```python
from build123d import *

# Parameters (mm, degrees)
SKETCH1_R           = 27.875
SKETCH1_R_2         = 17.875
BOSS_EXTRUDE1_DEPTH = 196.5
SKETCH2_R           = 11.53
CUT_EXTRUDE1_DEPTH  = 201.415271998


with BuildPart() as part:
    # Sketch1 → Boss-Extrude1 (new body)
    with BuildSketch(Plane(origin=(0, 0, 0), x_dir=(1, 0, 0), z_dir=(0, 1, 0))):
        with Locations(Location((0, 0, 0), (0, 0, 270))):
            Circle(SKETCH1_R)
        with Locations(Location((0, 0, 0), (0, 0, 270))):
            Circle(SKETCH1_R_2, mode=Mode.SUBTRACT)
    extrude(amount=BOSS_EXTRUDE1_DEPTH)

    # Sketch2 → Cut-Extrude1 (cut, through all)
    with BuildSketch(Plane(origin=(0, 0, 0), x_dir=(0, 0, -1), z_dir=(1, 0, 0))):
        with Locations((0, 131.8)):
            Circle(SKETCH2_R)
        with Locations((0, 80.8)):
            Circle(SKETCH2_R)
        with Locations((0, 29.8)):
            Circle(SKETCH2_R)
    extrude(amount=-CUT_EXTRUDE1_DEPTH, mode=Mode.SUBTRACT)


solid = part.part
```
Work out the finished part from the listing and answer in its coordinate system (mm). A direction names the side the tool comes from. Give positions to 0.01 mm unless a question says otherwise; leave off trailing zeros. Write each loop counter-clockwise with the first axis right and the second up, starting at its lowest first coordinate (ties: lowest second). Pieces come first, ordered by that corner, then holes.
(1) The part is cut by section B-B on x = 0. Write down the section's boundary in (y, z) (3 decimals).
Final values:
outline: (0, -27.875) - (196.5, -27.875) - (196.5, -17.875) - (0, -17.875) - close; (0, 17.875) - (196.5, 17.875) - (196.5, 27.875) - (0, 27.875) - close
(2) The part is cut by section D-D on z = -7.5. Write down the section's boundary in (x, y), plus the area to 3 significant figures.
Final values:
outline: (-26.85, 0) - (-16.23, 0) - (-16.23, 21.04) - (-26.85, 21.04) - close; (-26.85, 38.56) - (-16.23, 38.56) - (-16.23, 72.04) - (-26.85, 72.04) - close; (-26.85, 89.56) - (-16.23, 89.56) - (-16.23, 123.04) - (-26.85, 123.04) - close; (-26.85, 140.56) - (-16.23, 140.56) - (-16.23, 196.5) - (-26.85, 196.5) - close; (16.23, 0) - (26.85, 0) - (26.85, 196.5) - (16.23, 196.5) - close
area: 3,620 mm2
(3) Straight lines are drawn through the part: line 1 (Y direction, x = -18.75, z = 0); line 2 (X direction, y = 177, z = 1); line 3 (Z direction, x = -8.5, y = 85). For each, find the intervals that lie inside material, in ascending order.
Final values:
line 1: y = 0 to 18.27, 41.33 to 69.27, 92.33 to 120.27, 143.33 to 196.5
line 2: x = -27.86 to -17.85, 17.85 to 27.86
line 3: z = -26.55 to -15.72, 15.72 to 26.55
(4) Flat-ended cylindrical pins translate along their axes: pin 1 Ø12 at (x, y) = (-20, 167.5) entering from -Z; pin 2 Ø12 at (x, z) = (9, -17.5) entering from -Y; pin 3 Ø21 at (y, z) = (29.8, 0) entering from -X; pin 4 Ø18.5 at (y, z) = (131.8, 0) entering from -X. Find the tip coordinate at first contact, or state that the pin passes through.
Final values:
pin 1: stops at z = -24.1
pin 2: stops at y = 0
pin 3: stops at x = 14.47
pin 4: stops at x = 15.3
(5) The part is cut by section A-A on z = 0. Write down the section's boundary in (x, y) (3 decimals).
Final values:
outline: (-27.875, 0) - (-17.875, 0) - (-17.875, 18.27) - (-27.875, 18.27) - close; (-27.875, 41.33) - (-17.875, 41.33) - (-17.875, 69.27) - (-27.875, 69.27) - close; (-27.875, 92.33) - (-17.875, 92.33) - (-17.875, 120.27) - (-27.875, 120.27) - close; (-27.875, 143.33) - (-17.875, 143.33) - (-17.875, 196.5) - (-27.875, 196.5) - close; (17.875, 0) - (27.875, 0) - (27.875, 196.5) - (17.875, 196.5) - close
(6) The mould has two halves that part along X. Classify faces 3 (the flat face through (0.4, 196.5, 18.2)), 4 (the cylindrical face through (17.723, 96.874, -2.327)), 5 (the cylindrical face through (27.638, 96.874, -3.629)): pulls with the +X half, pulls with the -X half, needs draft (parallel to the pull), parting line crosses it, or undercut.
Final values:
face 3: needs draft
face 4: undercut
face 5: parting line crosses it
(7) The part is cut by section C-C on y = 52. Write down the section's boundary in (x, z) (3 decimals), plus the area to 3 significant figures.
Final values:
outline: circle Ø55.75 at (0, 0); hole circle Ø35.75 at (0, 0)
area: 1,440 mm2
(8) Which of the six approach directions +Z, -Z, +X, -X, +Y, -Y give full straight-line access (tool end or side, diameter ignored) to faces 1 (the cylindrical face through (-20.67, 135.26, -11)), 2 (the flat face through (0.4, 0, 18.2))?
Final values:
face 1: -X
face 2: +Z, -Z, +X, -X, -Y
